from build123d import *

# Parameters (mm, degrees)
SKETCH1_R           = 3.175
BOSS_EXTRUDE1_DEPTH = 31.75
SKETCH2_W           = 19.05
SKETCH2_H           = 25.4
SKETCH2_H_2         = 9.525
CUT_EXTRUDE1_DEPTH  = 19.05


with BuildPart() as part:
    # Sketch1 → Boss-Extrude1 (new body)
    with BuildSketch(Plane.XY):
        with BuildLine():
            Line((-9.525, 25.4), (-9.525, 0))
            ThreePointArc((-9.525, 0), (0, -9.525), (9.525, 0))
            Line((9.525, 0), (9.525, 3.175))
            Line((9.525, 3.175), (187.325, 3.175))
            ThreePointArc((187.325, 3.175), (196.85, 12.7), (187.325, 22.225))
            Line((187.325, 22.225), (9.525, 22.225))
            Line((9.525, 22.225), (9.525, 25.4))
            ThreePointArc((9.525, 25.4), (0, 34.925), (-9.525, 25.4))
        make_face()
        Circle(SKETCH1_R, mode=Mode.SUBTRACT)
        with Locations((0, 25.4)):
            Circle(SKETCH1_R, mode=Mode.SUBTRACT)
    extrude(amount=BOSS_EXTRUDE1_DEPTH)

    # Sketch2 → Cut-Extrude1 (cut)
    with BuildSketch(Plane.ZY.offset(9.525)):
        with Locations((15.875, 12.7)):
            Rectangle(SKETCH2_W, SKETCH2_H)
        with Locations((15.875, 30.1625)):
            Rectangle(SKETCH2_W, SKETCH2_H_2)
        with Locations((15.875, -4.7625)):
            Rectangle(SKETCH2_W, SKETCH2_H_2)
    extrude(amount=-CUT_EXTRUDE1_DEPTH, mode=Mode.SUBTRACT)


solid = part.part
CAD build for the part. Positions are in the model's coordinates, mm. A direction names the side the tool comes from. Round coordinates to 2 decimals unless told otherwise and drop trailing zeros. Write each loop counter-clockwise with the first axis right and the second up, starting at its lowest first coordinate (ties: lowest second). Pieces come first, ordered by that corner, then holes. Notation, with made-up numbers: M -8.75,-37.5 L 39.25,-37.5 A24 cw 39.25,-21.5 Z; hole C -25,-13.5 d7. An arc over 180 degrees is marked long. Put each result on its own line as item: value. Start each with the question number.
1) Saw through at B-B, the plane z = 27.5. Write the cut outline in (x, y) (3 decimals), and give its area (3 significant figures).
2) Drill centre lines: probe 1 along Y at (x, z) = (0, 3) (3 decimals); probe 2 along X at (y, z) = (25.4, 27) (3 decimals); probe 3 along Y at (x, z) = (107, 24.5) (3 decimals). Where is each one in solid material? Low to high. Write a range as [from, to].
3) Saw through at C-C, the plane y = 31. Write the cut outline in (x, z), and give its area (3 significant figures).
4) 3-axis set-ups, long thin cutter, end or side, ignore diameter. For faces 4 (the flat face through (0, 13, 6.35)), 5 (the cylindrical face through (-0.41, 28.55, 28.53)), 6 (the flat face through (100, 22.225, 16)), 7 (the flat face through (97, 3.175, 16)), 8 (the flat face through (-9.525, 13, 29)): which of +Z, -Z, +X, -X, +Y, -Y reach the whole face in a straight line?
5) Saw through at A-A, the plane x = 0. Write the cut outline in (y, z) (3 decimals), and give its area (3 significant figures).
6) Pull direction Y, two halves, no side cores. Call faces 1 (the flat face through (-9.525, 13, 3)), 2 (the cylindrical face through (-0.41, 28.55, 3.13)), 3 (the cylindrical face through (196.848, 12.491, 15.653)): pulls with the +Y half, pulls with the -Y half, needs draft (parallel to the pull), parting line crosses it, or undercut.
7) Saw through at D-D, the plane y = 12.7. Write the cut outline in (x, z) (3 decimals), and give its area (3 significant figures).
8) Pin check, flat tips, straight feed: pin 1 Ø2.5 at (y, z) = (1, 4) entering from +X (3 decimals); pin 2 Ø2 at (x, z) = (51.5, 14.5) entering from +Y (3 decimals); pin 3 Ø8 at (x, z) = (126, 17.5) entering from -Y (3 decimals); pin 4 Ø4 at (x, y) = (0, 25.4) entering from +Z. Stop position of each tip, or through.
Resolved:
1. outline: M -9.525,0 A9.525 ccw 9.525,0 L 9.525,3.175 L 187.325,3.175 A9.525 ccw 187.325,22.225 L 9.525,22.225 L 9.525,25.4 A9.525 ccw -9.525,25.4 Z; hole C 0,0 d6.35; hole C 0,25.4 d6.35
1. area: 4,240 mm²
2. probe 1: [-9.525, -3.175], [3.175, 22.225], [28.575, 34.925]
2. probe 2: [-9.525, -3.175], [3.175, 9.525]
2. probe 3: [3.175, 22.225]
3. outline: M -7.7,0 L 7.7,0 L 7.7,6.35 L -7.7,6.35 Z; M -7.7,25.4 L 7.7,25.4 L 7.7,31.75 L -7.7,31.75 Z
3. area: 196 mm²
4. face 4: -X, +Y, -Y
4. face 5: +Z, -Z
4. face 6: +Z, -Z, +X, +Y
4. face 7: +Z, -Z, +X, -Y
4. face 8: +Z, -Z, -X, +Y, -Y
5. outline: M -9.525,0 L -3.175,0 L -3.175,6.35 L -9.525,6.35 Z; M -9.525,25.4 L -3.175,25.4 L -3.175,31.75 L -9.525,31.75 Z; M 3.175,0 L 22.225,0 L 22.225,6.35 L 3.175,6.35 Z; M 3.175,25.4 L 22.225,25.4 L 22.225,31.75 L 3.175,31.75 Z; M 28.575,0 L 34.925,0 L 34.925,6.35 L 28.575,6.35 Z; M 28.575,25.4 L 34.925,25.4 L 34.925,31.75 L 28.575,31.75 Z
5. area: 403 mm²
6. face 1: needs draft
6. face 2: undercut
6. face 3: parting line crosses it
7. outline: M -9.525,0 L 196.85,0 L 196.85,31.75 L -9.525,31.75 L -9.525,25.4 L 9.525,25.4 L 9.525,6.35 L -9.525,6.35 Z
7. area: 6,190 mm²
8. pin 1: x = 9.525
8. pin 2: y = 22.225
8. pin 3: y = 3.175
8. pin 4: through
